Read the model definition and answer for the solid it produces. Units are mm, in the model's axes. Face numbers are marked on the shaded views. A direction names the side the tool comes from. Round coordinates to 2 decimals unless told otherwise and drop trailing zeros. Loops run counter-clockwise (first coordinate to the right, second up) from the corner with the lowest first, then second, coordinate; pieces in that order, holes last. Notation, with made-up numbers: (28.5, -34) - (40.5, -34) arc R37 cw to (40.5, 5) - close; hole circle Ø8 at (87.25, 59). An arc over 180 degrees is marked (long way). Use CSV: the item, a comma, the result in double quotes. Start each with the question number.
1. Find section A-A (y = 3). Give the vertices of the cut face in (x, z), and give its area (3 significant figures).
2. Find section B-B (y = 6). Give the vertices of the cut face in (x, z) (3 decimals).
3. A tool of negligible diameter and unlimited length cuts with its end or side. For the marked faces 1, 2 and 3, from which of +Z, -Z, +X, -X, +Y, -Y can it reach the whole face along a straight path? Write none if from no direction.
4. Find section C-C (z = 8). Give the vertices of the cut face in (x, y).
5. Given pin 1 Ø6 at (x, y) = (2, 14) entering from +Z; pin 2 Ø2 at (x, y) = (-7, 3) entering from +Z; pin 3 Ø4 at (x, z) = (9, 7.5) entering from +Y, each flat-ended and moving along its own axis, determine where each tip first touches the part or whether it passes through.
6. Determine the mould class of the marked faces 4, 5, 6 and 7 for opening direction Z: +Z half, -Z half, draft (parallel to the pull), parting line (faces both ways), or undercut.
7. Find section D-D (x = 0). Give the vertices of the cut face in (y, z), and give its area (3 significant figures).
8. Consider line 1 along Z through (x, y) = (10.5, 0.6); line 2 along X through (y, z) = (0.5, -10.4); line 3 along Z through (x, y) = (6, 3.75). Determine where each line is inside the solid, lowest interval first.
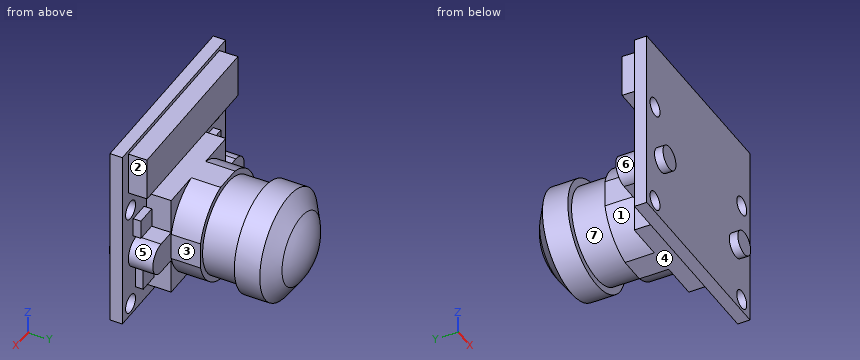
from build123d import *

# Parameters (mm, degrees)
ESQUISSE1_W        = 25
ESQUISSE1_H        = 24
BOSS_EXTRU_1_DEPTH = 1.6
BOSS_EXTRU_2_DEPTH = 3.18
BOSS_EXTRU_3_DEPTH = 3.8
ESQUISSE6_R        = 6.1
BOSS_EXTRU_4_DEPTH = 4.6
D_GAGEMENT_M21_D   = 2.4
ESQUISSE11_W       = 22
ESQUISSE11_H       = 5.6
BOSS_EXTRU_6_DEPTH = 2.4
ESQUISSE12_R       = 1.56
BOSS_EXTRU_7_DEPTH = 1.1
ESQUISSE13_W       = 2.577210691
ESQUISSE13_H       = 3.020616424
ESQUISSE13_W_2     = 2.628074632
ESQUISSE13_H_2     = 2.477608005
ESQUISSE13_W_3     = 2.260050421
ESQUISSE13_H_3     = 2.470679231
ESQUISSE13_W_4     = 2.751019587
ESQUISSE13_H_4     = 2.314618906
BOSS_EXTRU_8_DEPTH = 1


with BuildPart() as part:
    # Esquisse1 → Boss.-Extru.1 (new body)
    with BuildSketch(Plane(origin=(0, 0, 0), x_dir=(1, 0, 0), z_dir=(0, 1, 0))):
        Rectangle(ESQUISSE1_W, ESQUISSE1_H)
    extrude(amount=BOSS_EXTRU_1_DEPTH)

    # Esquisse4 → Boss.-Extru.2 (add)
    with BuildSketch(Plane(origin=(0, 1.6, 0), x_dir=(1, 0, 0), z_dir=(0, 1, 0))):
        with BuildLine():
            Line((6.6, 10.25), (6.6, 5.65))
            Line((6.6, 5.65), (9.05, 5.65))
            ThreePointArc((9.05, 5.65), (11.05, 3.65), (9.05, 1.65))
            Line((9.05, 1.65), (6.6, 1.65))
            Line((6.6, 1.65), (6.6, -2.95))
            Line((6.6, -2.95), (-6.6, -2.95))
            Line((-6.6, -2.95), (-6.6, 1.65))
            Line((-6.6, 1.65), (-9.05, 1.65))
            ThreePointArc((-9.05, 1.65), (-11.05, 3.65), (-9.05, 5.65))
            Line((-9.05, 5.65), (-6.6, 5.65))
            Line((-6.6, 5.65), (-6.6, 10.25))
            Line((-6.6, 10.25), (6.6, 10.25))
        make_face()
    extrude(amount=BOSS_EXTRU_2_DEPTH)

    # Esquisse5 → Boss.-Extru.3 (add)
    with BuildSketch(Plane(origin=(0, 4.78, 0), x_dir=(1, 0, 0), z_dir=(0, 1, 0))):
        with BuildLine():
            Line((-6.6, 1.912005466), (-6.6, 5.387994534))
            ThreePointArc((-6.6, 5.387994534), (-4.826003782, 8.476003782), (-1.737994534, 10.25))
            Line((-1.737994534, 10.25), (1.737994534, 10.25))
            ThreePointArc((1.737994534, 10.25), (4.826003782, 8.476003782), (6.6, 5.387994534))
            Line((6.6, 5.387994534), (6.6, 1.912005466))
            ThreePointArc((6.6, 1.912005466), (4.826003782, -1.176003782), (1.737994534, -2.95))
            Line((1.737994534, -2.95), (-1.737994534, -2.95))
            ThreePointArc((-1.737994534, -2.95), (-4.826003782, -1.176003782), (-6.6, 1.912005466))
        make_face()
    extrude(amount=BOSS_EXTRU_3_DEPTH)

    # Esquisse6 → Boss.-Extru.4 (add)
    with BuildSketch(Plane(origin=(0, 8.58, 0), x_dir=(1, 0, 0), z_dir=(0, 1, 0))):
        with Locations(Location((0, 3.65, 0), (0, 0, 270))):
            Circle(ESQUISSE6_R)
    extrude(amount=BOSS_EXTRU_4_DEPTH)

    # Esquisse8 → R_volution1 (revolve)
    with BuildSketch(Plane.XY.offset(-3.65), mode=Mode.PRIVATE) as r_volution1_sk:
        with BuildLine():
            Line((0, 13.18), (-7, 13.18))
            Line((-7, 13.18), (-7, 16.48))
            Line((-7, 16.48), (-4.631719117, 18.098501714))
            ThreePointArc((-4.631719117, 18.098501714), (-2.423943549, 19.163964644), (0, 19.53))
            Line((0, 19.53), (0, 13.18))
        make_face()
    revolve(r_volution1_sk.sketch.rotate(Axis((0, 13.18, -3.65), (0, 1, 0)), 180), axis=Axis((0, 13.18, -3.65), (0, 1, 0)))

    # D_gagement M21 (through all)
    with Locations(Plane(origin=(0, 1.6, 0), x_dir=(1, 0, 0), z_dir=(0, 1, 0))):
        with Locations((-10.5, 10.4), (10.5, 10.4), (10.5, -3.1), (-10.5, -3.1)):
            Hole(D_GAGEMENT_M21_D / 2)

    # Esquisse11 → Boss.-Extru.6 (add)
    with BuildSketch(Plane(origin=(0, 1.6, 0), x_dir=(1, 0, 0), z_dir=(0, 1, 0))):
        with Locations((0, -8.7)):
            Rectangle(ESQUISSE11_W, ESQUISSE11_H)
    extrude(amount=BOSS_EXTRU_6_DEPTH)

    # Esquisse12 → Boss.-Extru.7 (add)
    with BuildSketch(Plane.XZ):
        with Locations(Location((-9.05, -3.65, 0), (0, 0, 90))):
            Circle(ESQUISSE12_R)
        with Locations(Location((9.05, -3.65, 0), (0, 0, 90))):
            Circle(ESQUISSE12_R)
    extrude(amount=BOSS_EXTRU_7_DEPTH)

    # Esquisse13 → Boss.-Extru.8 (add)
    with BuildSketch(Plane(origin=(0, 1.6, 0), x_dir=(1, 0, 0), z_dir=(0, 1, 0))):
        with Locations((8.011394655, 7.289691788)):
            Rectangle(ESQUISSE13_W, ESQUISSE13_H)
        with Locations((8.546867327, -0.168124771)):
            Rectangle(ESQUISSE13_W_2, ESQUISSE13_H_2)
        with Locations((-8.36997479, -0.164660384)):
            Rectangle(ESQUISSE13_W_3, ESQUISSE13_H_3)
        with Locations((-8.324490207, 7.042690547)):
            Rectangle(ESQUISSE13_W_4, ESQUISSE13_H_4)
    extrude(amount=BOSS_EXTRU_8_DEPTH)


solid = part.part
Filled sheet:
1,outline,"(-11, 5.9) - (11, 5.9) - (11, 11.5) - (-11, 11.5) - close; (-9.05, -5.65) - (-6.6, -5.65) - (-6.6, -10.25) - (6.6, -10.25) - (6.6, -5.65) - (9.05, -5.65) arc R2 ccw to (9.05, -1.65) - (6.6, -1.65) - (6.6, 2.95) - (-6.6, 2.95) - (-6.6, -1.65) - (-9.05, -1.65) arc R2 ccw to start"
1,area,"330 mm²"
2,outline,"(-6.6, -5.388) arc R6.825 ccw to (-1.738, -10.25) - (1.738, -10.25) arc R6.825 ccw to (6.6, -5.388) - (6.6, -1.912) arc R6.825 ccw to (1.738, 2.95) - (-1.738, 2.95) arc R6.825 ccw to (-6.6, -1.912) - close"
3,face 1,"-Z, -X"
3,face 2,"+Z, +X, +Y"
3,face 3,"+Z, -Z, +X"
4,outline,"(-12.5, 0) - (12.5, 0) - (12.5, 1.6) - (11, 1.6) - (11, 4) - (-11, 4) - (-11, 1.6) - (-12.5, 1.6) - close"
5,pin 1,"stops at z = 3.35"
5,pin 2,"stops at z = 11.5"
5,pin 3,"stops at y = 4"
6,face 4,"-Z half"
6,face 5,"undercut"
6,face 6,"undercut"
6,face 7,"parting line"
7,outline,"(0, -12) - (1.6, -12) - (1.6, -10.25) - (8.58, -10.25) - (8.58, -9.75) - (13.18, -9.75) - (13.18, -10.65) - (16.48, -10.65) - (18.1, -8.28) arc R8.21 ccw to (18.1, 0.98) - (16.48, 3.35) - (13.18, 3.35) - (13.18, 2.45) - (8.58, 2.45) - (8.58, 2.95) - (1.6, 2.95) - (1.6, 5.9) - (4, 5.9) - (4, 11.5) - (1.6, 11.5) - (1.6, 12) - (0, 12) - close"
7,area,"274 mm²"
8,line 1,"z = -12 to -11.6, -9.2 to 1.9, 4.3 to 12"
8,line 2,"x = -12.5 to -11.7, -9.3 to 9.3, 11.7 to 12.5"
8,line 3,"z = -10.25 to 2.95, 5.9 to 11.5"
